Autodesk Inventor part; units mm, degrees
ref_plane "Начальная плоскость" through (0, 0, -25) normal (0, 0, 1) x (1, 0, 0)
ref_plane "Конечная плоскость" through (0, 0, 1025) normal (0, 0, 1) x (1, 0, 0)
ref_plane "РабПлоскость4" through (0, 0, -25) normal (0.7071, 0, -0.7071) x (-0.7071, 0, -0.7071)
ref_plane "Начальная плоскость" through (0, 0, -25) normal (0, 0, 1) x (1, 0, 0)
ref_plane "Конечная плоскость" through (0, 0, 1025) normal (0, 0, 1) x (1, 0, 0)
sketch "Эскиз" plane through (0, 0, 0) normal (0, 0, 1) x (1, 0, 0)
  line L0 (0, 0) -> (0, 50)
  line L1 (0, 50) -> (50, 50)
  line L2 (50, 50) -> (50, 47.6544)
  line L3 (45.8589, 43.1687) -> (13.8222, 40.6058)
  line L4 (6, 32.1328) -> (6, 0)
  line L5 (6, 0) -> (0, 0) construction
  line L6 (25, 50) -> (25, 41.5) construction
  line L7 (50, 43.5) -> (50, 41.5) construction
  line L8 (50, 41.5) -> (25, 41.5) construction
  line L9 (0, 15) -> (0, -27) construction
  line L10 (-5.539, 0) -> (16.0067, 0) construction
  line L11 (0, 0) -> (0, -50)
  line L12 (0, -50) -> (50, -50)
  line L13 (50, -50) -> (50, -47.6544)
  line L14 (45.8589, -43.1687) -> (13.8222, -40.6058)
  line L15 (6, -32.1328) -> (6, 0)
  arc A0 (13.8222, 40.6058) -> (6, 32.1328) centre (14.5, 32.1328) ccw
  arc A1 (6, -32.1328) -> (13.8222, -40.6058) centre (14.5, -32.1328) ccw
  arc A2 (45.8589, 43.1687) -> (50, 47.6544) centre (45.5, 47.6544) ccw
  arc A3 (50, -47.6544) -> (45.8589, -43.1687) centre (45.5, -47.6544) ccw
  line L16 (0, 70) -> (0, -70) construction
  line L17 (-16.8222, 0) -> (62.1602, 0) construction
  point P0 (6, 39.98)
  point P1 (50, -43.5)
  point P2 (6, -39.98)
  point P3 (25, -50)
  point P4 (25, -41.5)
  dimension "d0" = 6
  dimension "d1" = 50
  dimension "d2" = 50
  dimension "d3" = 8.5
  dimension "d4" = 25
  dimension "d5" = 2
  dimension "d23" = 8.5
  dimension "d24" = 4.5
  dimension "d25" = 0
extrude "Тело" add sketch "Эскиз" along normal up to surface (1050 mm away) from surface at -25
sketch "Sketch3" plane through (0, 0, 0) normal (0, 0, 1) x (1, 0, 0)
  line L0 (0, 0) -> (10, 0)
ref_plane "Work Plane3" through (0, 0, 0) normal (0, -1, 0) x (1, 0, 0)
sketch "Sketch4" plane through (0, 0, 0) normal (0, -1, 0) x (1, 0, 0)
  line L0 (-2, -25) -> (12, -25)
  line L1 (-2, 1025) -> (12, 1025)
  dimension "d29" = 1050
ref_plane "РабПлоскость4" through (0, 0, -25) normal (0.7071, 0, -0.7071) x (-0.7071, 0, -0.7071)
split "Разделение1" plane through (0, 0, -25) removes the side toward (0.7071, 0, -0.7071)
ref_plane "РабПлоскость5" through (0, 0, 1025) normal (0.7071, 0, 0.7071) x (0.7071, 0, -0.7071)
split "Разделение2" plane through (0, 0, 1025) removes the side toward (0.7071, 0, 0.7071)
equation "\"d0\" = G_T"
equation "\"d1\" = 0.5 * G_H"
equation "\"d2\" = G_W"
equation "\"d3\" = G_T1"
equation "\"d4\" = G_C"
equation "\"d23\" = G_IR"
equation "\"d24\" = G_ER"
equation "\"d6\" = G_L"
equation "\"G_W\" = 50"
equation "\"G_T\" = 6"
equation "\"G_T1\" = 8.5"
equation "\"G_NG\" = 0.08"
equation "\"G_ER\" = 4.5"
equation "\"G_IR\" = 8.5"
equation "\"G_C\" = 25"
equation "\"G_L\" = d29"
equation "\"ex\" = 0"
equation "\"G_OFFSET_START\" = 25"
equation "\"G_OFFSET_END\" = 25"
equation "\"d26\" = -G_OFFSET_START"
equation "\"d27\" = G_OFFSET_END + B_L"
properties part number "DIN1026 - U 100 - 1050" material "Сталь, углеродистая"
Read the model definition and answer for the solid it produces. Units are mm, in the model's axes. A direction names the side the tool comes from. Give positions to 0.01 mm unless a question says otherwise; leave off trailing zeros. Order: outer loops, then holes, each group sorted by start corner. A loop starts at its lowest first (then second) coordinate and runs counter-clockwise, first axis right, second up.
(1) Find section C-C (y = -10). Give the vertices of the cut face in (x, z).
(2) For a pull along Y with two mould halves and no side action, classify faces 1 (the flat face through (30.065, 41.905, 492.844)), 2 (the flat face through (5, 0, 1020)), 3 (the flat face through (25, -50, 493)), 4 (the flat face through (25, 50, 493)) as released by +Y, released by -Y, zero draft, split by the parting line, or undercut.
(3) Find section B-B (z = 942). Give the vertices of the cut face in (x, y).
(4) Find section A-A (x = 34.5). Give the vertices of the cut face in (y, z).
(5) Straight lines are drawn through the part: L1, parallel to Y at x = 13.5, z = 377; L2, parallel to Y at x = 16, z = 922; L3, parallel to X at y = 1, z = 783.5. For each, find the intervals that lie inside material, in ascending order.
(6) For faces 5 (the flat face through (30.065, -41.905, 492.844)), 6 (the flat face through (5, 0, -20)), determine the directions among +Z, -Z, +X, -X, +Y, -Y from which every point of the face is accessible in a straight line to the end or side of a thin tool.
Result sheet:
1. outline: (0, -25) - (6, -19) - (6, 1019) - (0, 1025) - close
2. face 1: undercut
2. face 2: zero draft
2. face 3: released by -Y
2. face 4: released by +Y
3. outline: (0, -50) - (50, -50) - (50, -47.65) arc R4.5 ccw to (45.86, -43.17) - (13.82, -40.61) arc R8.5 cw to (6, -32.13) - (6, 32.13) arc R8.5 cw to (13.82, 40.61) - (45.86, 43.17) arc R4.5 ccw to (50, 47.65) - (50, 50) - (0, 50) - close
4. outline: (-50, 9.5) - (-42.26, 9.5) - (-42.26, 990.5) - (-50, 990.5) - close; (42.26, 9.5) - (50, 9.5) - (50, 990.5) - (42.26, 990.5) - close
5. L1: y = -50 to -40.57, 40.57 to 50
5. L2: y = -50 to -40.78, 40.78 to 50
5. L3: x = 0 to 6
6. face 5: +Z, -Z, +X
6. face 6: -Z, +X, +Y, -Y
